from build123d import *

# Parameters (mm, degrees)
F0_W     = 355.6
F0_H     = 88.9
F1_DEPTH = 9.525
F3_DEPTH = 3.175
F5_DEPTH = 19.05


# Not quite as in the source:
# - a pattern or mirror of a feature is missing from the dataset's text; its kind, count and spacing are read off the source's solid


with BuildPart() as f1:
    # F0 (on Front) → F1 (new body, symmetric)
    with BuildSketch(Plane.XZ):
        Rectangle(F0_W, F0_H)
    extrude(amount=F1_DEPTH, both=True)

    # F2 (on Front) → F3 (join, symmetric)
    with BuildSketch(Plane.XZ):
        Polygon((-177.8, -31.75), (-177.8, 44.45), (-190.5, 44.45), (-190.5, 31.75), (-203.2, 31.75), (-203.2, -31.75), align=None)
    f3 = extrude(amount=F3_DEPTH, both=True)

    # F3_copies: F3 across plane
    add(f3.mirror(Plane(origin=(0, 0, 0), x_dir=(0, 0, 1), z_dir=(1, 0, 0))))

    # F4 (on face) → F5 (cut, through all)
    with BuildSketch(Plane.XZ.offset(9.525)):
        with BuildLine():
            ThreePointArc((146.05, -44.45), (0, -19.05), (-146.05, -44.45))
            Line((-146.05, -44.45), (146.05, -44.45))
        make_face()
    extrude(amount=-F5_DEPTH, mode=Mode.SUBTRACT)


solid = f1.part
Can you work these out from the model? Positions are in its coordinate system, mm. A direction names the side the tool comes from. Give positions to 0.01 mm unless a question says otherwise; leave off trailing zeros. Write each loop counter-clockwise with the first axis right and the second up, starting at its lowest first coordinate (ties: lowest second). Pieces come first, ordered by that corner, then holes. Notation, with made-up numbers: (51, 24.25) -> (81, 24.25) arc R17 cw to (81, 42.25) -> close; hole circle Ø7 at (-1.75, 21). An arc over 180 degrees is marked (long way). Answer as a JSON object with one key per item and string values. Group by question number.
Item 1: Suppose I cut it at B-B (z = 26.5). Please give me the cut outline in (x, y) (3 decimals), plus the area to 3 significant figures.
Item 2: Suppose I cut it at D-D (x = 31). Please give me the cut outline in (y, z) (3 decimals), plus the area to 3 significant figures.
Item 3: We'd pull the mould along X, two halves only. Please class faces 1 (the face through (-3, 0, 44.45)), 2 (the face through (-190.5, 0, 38)), 3 (the face through (2.086, -0.133, -19.055)): +X half, -X half, draft (parallel to the pull), parting line (faces both ways), or undercut.
Item 4: For faces 4 (the face through (191, 3.175, 7)), 5 (the face through (-191, -3.175, 7)), 6 (the face through (-191, 3.175, 7)), 7 (the face through (191, -3.175, 7)), 8 (the face through (190.5, 0, 38)), which set-ups out of +Z, -Z, +X, -X, +Y, -Y let a thin tool reach every point of the face, with its end or its side?
Item 5: I'm going to push flat-ended pins straight in: P1, Ø3, axis at x = 195.5, y = 0.5, coming from the +Z side; P2, Ø1.5, axis at y = -4, z = 8, coming from the +X side; P3, Ø8, axis at x = -104, y = 2, coming from the -Z side; P4, Ø6, axis at y = 4, z = 32, coming from the -X side. Where does each tip first touch, or does it pass through?
Item 6: Suppose I cut it at A-A (z = -26). Please give me the cut outline in (x, y) (3 decimals).
Item 7: Please list where these lines run through material, in increasing order: line 1 (X direction, y = 6.5, z = -2); line 2 (X direction, y = 0.75, z = 33.5); line 3 (Z direction, x = -119, y = -8.5). Write a range as [from, to].
Item 8: Suppose I cut it at C-C (x = -130.5). Please give me the cut outline in (y, z) (3 decimals).
Findings:
{
 "1": {"outline": "(-203.2, -3.175) -> (-177.8, -3.175) -> (-177.8, -9.525) -> (177.8, -9.525) -> (177.8, -3.175) -> (203.2, -3.175) -> (203.2, 3.175) -> (177.8, 3.175) -> (177.8, 9.525) -> (-177.8, 9.525) -> (-177.8, 3.175) -> (-203.2, 3.175) -> close", "area": "7,100 mm²"},
 "2": {"outline": "(-9.525, -20.162) -> (9.525, -20.162) -> (9.525, 44.45) -> (-9.525, 44.45) -> close", "area": "1,230 mm²"},
 "3": {"face 1": "draft", "face 2": "-X half", "face 3": "undercut"},
 "4": {"face 4": "+Z, -Z, +X, +Y", "face 5": "+Z, -Z, -X, -Y", "face 6": "+Z, -Z, -X, +Y", "face 7": "+Z, -Z, +X, -Y", "face 8": "+Z, +X, +Y, -Y"},
 "5": {"P1": "stops at z = 31.75", "P2": "stops at x = 177.8", "P3": "stops at z = -32.75", "P4": "stops at x = -203.2"},
 "6": {"outline": "(-203.2, -3.175) -> (-177.8, -3.175) -> (-177.8, -9.525) -> (-77.232, -9.525) -> (-77.232, 9.525) -> (-177.8, 9.525) -> (-177.8, 3.175) -> (-203.2, 3.175) -> close; (77.232, -9.525) -> (177.8, -9.525) -> (177.8, -3.175) -> (203.2, -3.175) -> (203.2, 3.175) -> (177.8, 3.175) -> (177.8, 9.525) -> (77.232, 9.525) -> close"},
 "7": {"line 1": "x = [-177.8, 177.8]", "line 2": "x = [-190.5, 190.5]", "line 3": "z = [-35.74, 44.45]"},
 "8": {"outline": "(-9.525, -39.203) -> (9.525, -39.203) -> (9.525, 44.45) -> (-9.525, 44.45) -> close"}
}
